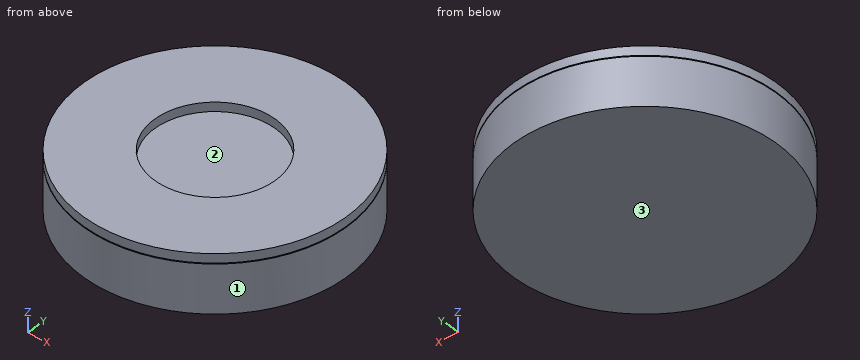
from build123d import *

# Parameters (mm, degrees)
SKIZZE2_R         = 72.5
BASE_DEPTH        = 32
SKIZZE3_W         = 1
SKIZZE3_H         = 0.5
SKIZZE4_R         = 33.25
LIDAR_SPACE_DEPTH = 5


with BuildPart() as part:
    # Skizze2 → Base (new body)
    with BuildSketch(Plane.XY):
        Circle(SKIZZE2_R)
    extrude(amount=BASE_DEPTH)

    # Skizze3 → Cover Seam (revolve, cut)
    with BuildSketch(Plane(origin=(0, 0, 0), x_dir=(1, 0, 0), z_dir=(0, 1, 0)), mode=Mode.PRIVATE) as cover_seam_sk:
        with Locations((72, -26.75)):
            Rectangle(SKIZZE3_W, SKIZZE3_H)
    revolve(cover_seam_sk.sketch.rotate(Axis((0, 0, 0), (0, 0, 1)), 180), axis=Axis((0, 0, 0), (0, 0, 1)), mode=Mode.SUBTRACT)

    # Skizze4 → Lidar Space (cut)
    with BuildSketch(Plane.XY.offset(32)):
        Circle(SKIZZE4_R)
    extrude(amount=-LIDAR_SPACE_DEPTH, mode=Mode.SUBTRACT)


solid = part.part
Build history of the part. All positions in model axes, mm. Face numbers are marked on the shaded views. Coordinates: 2 decimals unless noted, no trailing zeros. Order: outer loops, then holes, each group sorted by start corner. A loop starts at its lowest first (then second) coordinate and runs counter-clockwise, first axis right, second up. Notation, with made-up numbers: M 89,41.25 L 103,41.25 A25 cw 103,66.25 Z; hole C 88.25,29.25 d10. An arc over 180 degrees is marked long. One line per question, with ' | ' between items. Start each with the question number.
Q1. Two-plate mould, pull along X, no slides. Class the marked faces 1, 2 and 3: +X half, -X half, draft (parallel to the pull), parting line (faces both ways), or undercut.
Q2. Saw through at C-C (z = 24). List the corners of the cut face in (x, y).
Q3. Flat gauge pins, fed straight in: pin 1 Ø5 at (y, z) = (-20.5, 21.5) entering from +X; pin 2 Ø8 at (x, z) = (-23, 15.5) entering from +Y; pin 3 Ø4 at (y, z) = (-29, 19) entering from -X. Where does each tip first touch, or does it go through?
Q4. Saw through at A-A (y = 0). List the corners of the cut face in (x, z).
Q5. Saw through at D-D (y = -59). List the corners of the cut face in (x, z), then the cut area to 3 significant figures.
Q6. Probe L1, parallel to Y at x = 0, z = 30; L2, parallel to Y at x = 55.5, z = 13; L3, parallel to Y at x = -30.5, z = 4. List the from-to ranges inside material, lowest first. Write a range as from..to.
Check values:
1) face 1: parting line | face 2: undercut | face 3: draft
2) outline: C 0,0 d145
3) pin 1: stops at x = 70.23 | pin 2: stops at y = 69.97 | pin 3: stops at x = -67.28
4) outline: M -72.5,0 L 72.5,0 L 72.5,26.5 L 71.5,26.5 L 71.5,27 L 72.5,27 L 72.5,32 L 33.25,32 L 33.25,27 L -33.25,27 L -33.25,32 L -72.5,32 L -72.5,27 L -71.5,27 L -71.5,26.5 L -72.5,26.5 Z
5) outline: M -42.13,0 L 42.13,0 L 42.13,26.5 L 40.39,26.5 L 40.39,27 L 42.13,27 L 42.13,32 L -42.13,32 L -42.13,27 L -40.39,27 L -40.39,26.5 L -42.13,26.5 Z | area: 2,690 mm2
6) L1: y = -72.5..-33.25, 33.25..72.5 | L2: y = -46.65..46.65 | L3: y = -65.77..65.77
